Geometry: final body of the model. Coordinates: model frame, mm. A direction names the side the tool comes from. Give positions to 0.01 mm unless a question says otherwise; leave off trailing zeros. Write each loop counter-clockwise with the first axis right and the second up, starting at its lowest first coordinate (ties: lowest second). Pieces come first, ordered by that corner, then holes. Notation, with made-up numbers: M -33.75,26.25 L 2.25,26.25 A9 cw 2.25,32.25 Z; hole C -27,5.5 d10. An arc over 180 degrees is marked long. Use a Markdown table: item, result. Add a question column.
1) Line query: line 1 (Y direction, x = 22.5, z = -90); line 2 (X direction, y = 109.5, z = -88); line 3 (Z direction, x = 5, y = 24). Output: solid intervals per line, ascending.
2) Section C-C on y = 165. Return the cut outline in (x, z), then the cut area to 3 significant figures.
3) Draft query along X for faces 4 (the flat face through (96, 56, -7.62)), 5 (the flat face through (51, 121.755, -96)). Return one class per face: +X half, -X half, draft (parallel to the pull), parting line (faces both ways), or undercut.
4) Section A-A on z = -24. Return the cut outline in (x, y) (3 decimals).
5) Section B-B on x = 84. Return the cut outline in (y, z) (3 decimals), then the cut area to 3 significant figures.
6) Set-up query: faces 1 (the flat face through (4, 170, -7.62)), 2 (the flat face through (49, 119, -7.62)), 3 (the flat face through (51, 116.675, -96)). Return all of +Z, -Z, +X, -X, +Y, -Y with unobstructed straight access to the full face (end or side cutting, diameter ignored); none if empty.
```python
from build123d import *

# Parameters (mm, degrees)
SKETCH1_W           = 100
SKETCH1_H           = 100
BOSS_EXTRUDE1_DEPTH = 227
SKETCH6_W           = 84.76
SKETCH6_H           = 97.625
SKETCH6_H_2         = 6.35
CUT_EXTRUDE3_DEPTH  = 268.44906057
SKETCH10_W          = 84.76
SKETCH10_H          = 97.625
SKETCH10_H_2        = 6.35
CUT_EXTRUDE4_DEPTH  = 268.44906057
SKETCH11_W          = 84.76
SKETCH11_H          = 84.76
CUT_EXTRUDE5_DEPTH  = 25.4


with BuildPart() as part:
    # Sketch1 → Boss-Extrude1 (new body)
    with BuildSketch(Plane(origin=(0, 0, 0), x_dir=(1, 0, 0), z_dir=(0, 1, 0))):
        with Locations((50, 50)):
            Rectangle(SKETCH1_W, SKETCH1_H)
    extrude(amount=BOSS_EXTRUDE1_DEPTH)

    # Sketch6 → Cut-Extrude3 (cut, through all)
    with BuildSketch(Plane(origin=(100, 0, 0), x_dir=(0, 0, -1), z_dir=(1, 0, 0))):
        with Locations((50, 56.4325)):
            Rectangle(SKETCH6_W, SKETCH6_H)
        with Locations((50, 113.5)):
            Rectangle(SKETCH6_W, SKETCH6_H_2)
        with Locations((50, 170.5675)):
            Rectangle(SKETCH6_W, SKETCH6_H)
    extrude(amount=-CUT_EXTRUDE3_DEPTH, mode=Mode.SUBTRACT)

    # Sketch10 → Cut-Extrude4 (cut, through all)
    with BuildSketch(Plane.XY):
        with Locations((50, 170.5675)):
            Rectangle(SKETCH10_W, SKETCH10_H)
        with Locations((50, 113.5)):
            Rectangle(SKETCH10_W, SKETCH10_H_2)
        with Locations((50, 56.4325)):
            Rectangle(SKETCH10_W, SKETCH10_H)
    extrude(amount=-CUT_EXTRUDE4_DEPTH, mode=Mode.SUBTRACT)

    # Sketch11 → Cut-Extrude5 (cut)
    with BuildSketch(Plane(origin=(0, 121.755, 0), x_dir=(1, 0, 0), z_dir=(0, 1, 0))):
        with Locations((50, 50)):
            Rectangle(SKETCH11_W, SKETCH11_H)
    extrude(amount=-CUT_EXTRUDE5_DEPTH, mode=Mode.SUBTRACT)


solid = part.part
```
Found:
| question | item | result |
|---|---|---|
| 1 | line 1 | 0 to 7.62, 219.38 to 227 |
| 1 | line 2 | 0 to 7.62, 92.38 to 100 |
| 1 | line 3 | -100 to -92.38, -7.62 to 0 |
| 2 | outline | M 0,-100 L 7.62,-100 L 7.62,-92.38 L 0,-92.38 Z; M 0,-7.62 L 7.62,-7.62 L 7.62,0 L 0,0 Z; M 92.38,-100 L 100,-100 L 100,-92.38 L 92.38,-92.38 Z; M 92.38,-7.62 L 100,-7.62 L 100,0 L 92.38,0 Z |
| 2 | area | 232 mm² |
| 3 | face 4 | draft |
| 3 | face 5 | undercut |
| 4 | outline | M 0,0 L 100,0 L 100,7.62 L 0,7.62 Z; M 0,105.245 L 7.62,105.245 L 7.62,110.325 L 0,110.325 Z; M 0,116.675 L 7.62,116.675 L 7.62,121.755 L 0,121.755 Z; M 0,219.38 L 100,219.38 L 100,227 L 0,227 Z; M 92.38,105.245 L 100,105.245 L 100,110.325 L 92.38,110.325 Z; M 92.38,116.675 L 100,116.675 L 100,121.755 L 92.38,121.755 Z |
| 5 | outline | M 0,-100 L 7.62,-100 L 7.62,0 L 0,0 Z; M 105.245,-100 L 110.325,-100 L 110.325,-92.38 L 105.245,-92.38 Z; M 105.245,-7.62 L 110.325,-7.62 L 110.325,0 L 105.245,0 Z; M 116.675,-100 L 121.755,-100 L 121.755,-92.38 L 116.675,-92.38 Z; M 116.675,-7.62 L 121.755,-7.62 L 121.755,0 L 116.675,0 Z; M 219.38,-100 L 227,-100 L 227,0 L 219.38,0 Z |
| 5 | area | 1,680 mm² |
| 6 | face 1 | +X, -X |
| 6 | face 2 | none |
| 6 | face 3 | +Z, -Z |
